```python
from build123d import *

# Parameters (mm, degrees)
BOSS_EXTRUDE1_DEPTH = 50
SKETCH2_R           = 5
CUT_EXTRUDE1_DEPTH  = 477
BOSS_EXTRUDE2_DEPTH = 200


with BuildPart() as part:
    # Sketch1 → Boss-Extrude1 (new body)
    with BuildSketch(Plane.XY):
        Polygon((200, 32.5), (215, 32.5), (215, -32.5), (-215, -32.5), (-215, 32.5), (-200, 32.5), (-200, -17.5), (200, -17.5), align=None)
    extrude(amount=BOSS_EXTRUDE1_DEPTH)

    # Sketch2 → Cut-Extrude1 (cut)
    with BuildSketch(Plane(origin=(215, 0, 0), x_dir=(0, 0, -1), z_dir=(1, 0, 0))):
        with Locations((-25, 12.5)):
            Circle(SKETCH2_R)
    extrude(amount=-CUT_EXTRUDE1_DEPTH, mode=Mode.SUBTRACT)

    # Sketch3 → Boss-Extrude2 (add, symmetric)
    with BuildSketch(Plane(origin=(0, 0, 0), x_dir=(0, 0, -1), z_dir=(1, 0, 0))):
        Polygon((-50, -32.5), (-100, -46.367513459), (-50, -17.5), align=None)
    extrude(amount=BOSS_EXTRUDE2_DEPTH, both=True)


solid = part.part
```
Geometry check sheet. Reference: the model listing, model coordinates, mm. A direction names the side the tool comes from. Coordinates: 2 decimals unless noted, no trailing zeros. Order: outer loops, then holes, each group sorted by start corner. A loop starts at its lowest first (then second) coordinate and runs counter-clockwise, first axis right, second up.
Item 1: Section check A-A (z = 25). Enter the section's corners in (x, y).
Item 2: Section check B-B (y = 12.5). Enter the section's corners in (x, z), plus the area to 3 significant figures.
Item 3: Depth check by flat-ended pin: pin 1 (14.5 mm diameter, centred on y = -26, z = 64.5, fed in from -X); pin 2 (6 mm diameter, centred on y = 12.5, z = 25, fed in from -X); pin 3 (16.5 mm diameter, centred on x = -205, y = -2.5, fed in from +Z); pin 4 (8 mm diameter, centred on x = 107, z = 73, fed in from +Y). Enter the tip coordinate at first touch or a pass-through.
Item 4: Section check D-D (x = -189). Enter the section's corners in (y, z).
Item 5: Tool access check on faces 1 (the flat face through (3, -32.5, 25)), 2 (the flat face through (200, -32, 66)), 3 (the flat face through (-200, 2, 25)). Record the directions out of +Z, -Z, +X, -X, +Y, -Y that give a thin tool (end or side, any length) a straight path to the whole face; none if there is none.
Item 6: Scan lines: line 1 along X through (y, z) = (23, 13); line 2 along Z through (x, y) = (-203, 12); line 3 along Y through (x, z) = (211.75, 25). Record each from-to range of solid material in increasing order.
Item 7: Mould release check, pull along X, two halves, no side actions. Record for faces 4 (the flat face through (200, 7, 25)), 5 (the flat face through (208, 0, 50)), 6 (the flat face through (-200, -32, 66)): released by +X, released by -X, zero draft, split by the parting line, or undercut.
Item 8: Section check C-C (z = 42.5). Enter the section's corners in (x, y).
Check sheet entries:
1. outline: (-215, -32.5) - (215, -32.5) - (215, 7.5) - (200, 7.5) - (200, -17.5) - (-200, -17.5) - (-200, 7.5) - (-215, 7.5) - close; (-215, 17.5) - (-200, 17.5) - (-200, 32.5) - (-215, 32.5) - close; (200, 17.5) - (215, 17.5) - (215, 32.5) - (200, 32.5) - close
2. outline: (-215, 0) - (-200, 0) - (-200, 20) - (-215, 20) - close; (-215, 30) - (-200, 30) - (-200, 50) - (-215, 50) - close; (200, 0) - (215, 0) - (215, 20) - (200, 20) - close; (200, 30) - (215, 30) - (215, 50) - (200, 50) - close
2. area: 1,200 mm2
3. pin 1: stops at x = -200
3. pin 2: passes through
3. pin 3: stops at z = 50
3. pin 4: stops at y = -28.47
4. outline: (-46.37, 100) - (-32.5, 50) - (-32.5, 0) - (-17.5, 0) - (-17.5, 50) - close
5. face 1: -Z, +X, -X, -Y
5. face 2: +Z, +X, +Y, -Y
5. face 3: +Z, -Z, +Y
6. line 1: x = -215 to -200, 200 to 215
6. line 2: z = 0 to 20.03, 29.97 to 50
6. line 3: y = -32.5 to 7.5, 17.5 to 32.5
7. face 4: undercut
7. face 5: zero draft
7. face 6: released by -X
8. outline: (-215, -32.5) - (215, -32.5) - (215, 32.5) - (200, 32.5) - (200, -17.5) - (-200, -17.5) - (-200, 32.5) - (-215, 32.5) - close
